Autodesk Inventor part; units mm, degrees
ref_plane "YZ Plane" through (0, 0, 0) normal (1, 0, 0) x (0, 1, 0)
ref_plane "XZ Plane" through (0, 0, 0) normal (0, 1, 0) x (-1, 0, 0)
ref_plane "XY Plane" through (0, 0, 0) normal (0, 0, 1) x (1, 0, 0)
sketch "Sketch1" plane through (0, 0, 0) normal (0, 0, 1) x (1, 0, 0)
  line L0 (0, 0) -> (97, 0)
  line L1 (97, 0) -> (97, 65)
  line L2 (97, 65) -> (0, 65)
  line L3 (0, 65) -> (0, 0)
  circle A0 centre (48.5, 32.5) radius 3
  line L4 (63.5, 47.5) -> (61.5, 47.5)
  line L5 (61.5, 47.5) -> (61.5, 17.5)
  line L6 (61.5, 17.5) -> (63.5, 17.5)
  line L7 (63.5, 17.5) -> (63.5, 47.5)
  line L8 (33.5, 47.5) -> (35.5, 47.5)
  line L9 (35.5, 47.5) -> (35.5, 17.5)
  line L10 (35.5, 17.5) -> (33.5, 17.5)
  line L11 (33.5, 17.5) -> (33.5, 47.5)
  line L12 (35.5, 49.5718) -> (61.5, 49.5718)
  line L13 (61.5, 49.5718) -> (61.5, 47.5718)
  line L14 (61.5, 47.5718) -> (35.5, 47.5718)
  line L15 (35.5, 47.5718) -> (35.5, 49.5718)
  line L16 (48.5, 32.5) -> (31.2053, 32.5)
  line L17 (31.2053, 32.5) -> (48.5, 32.5)
  line L18 (48.5, 32.5) -> (67.3058, 32.5)
  line L19 (35.5, 15.4282) -> (61.5, 15.4282)
  line L20 (61.5, 17.4282) -> (35.5, 17.4282)
  line L21 (61.5, 15.4282) -> (61.5, 17.4282)
  line L22 (35.5, 15.4282) -> (35.5, 17.4282)
  point P0 (0, 32.5)
  point P1 (62.5, 47.5)
  dimension "d2" = 97
  dimension "d3" = 65
  dimension "d4" = 6
  dimension "d6" = 32.5
  dimension "d7" = 48.5
  dimension "d8" = 2
  dimension "d9" = 30
  dimension "d12" = 15
  dimension "d13" = 2
  dimension "d14" = 30
  dimension "d15" = 15
  dimension "d16" = 2
  dimension "d20" = 26
  dimension "d21" = 0
extrude "Extrusion1" add sketch "Sketch1" along normal mid plane 1.8
Geometry check sheet. Reference: the model listing, model coordinates, mm. A direction names the side the tool comes from. Give positions to 0.01 mm unless a question says otherwise; leave off trailing zeros. Loops run counter-clockwise (first coordinate to the right, second up) from the corner with the lowest first, then second, coordinate; pieces in that order, holes last. Notation, with made-up numbers: M 55.25,-6 L 98.25,-6 A20 ccw 98.25,19 Z; hole C -19.75,54 d2. An arc over 180 degrees is marked long. Write item = value, one per line.
(1) Sectioned sample at A-A, the plane y = 28. Record the cut outline in (x, z).
Answer below:
outline = M 0,-0.9 L 33.5,-0.9 L 33.5,0.9 L 0,0.9 Z; M 35.5,-0.9 L 61.5,-0.9 L 61.5,0.9 L 35.5,0.9 Z; M 63.5,-0.9 L 97,-0.9 L 97,0.9 L 63.5,0.9 Z
(2) Release check for a two-part mould opening along X. For faces 1 (the face through (61.5, 49, 0)), 2 (the face through (0, 33, 0)), 3 (the face through (48, 0, 0)) record: released by +X, released by -X, zero draft, split by the parting line, or undercut.
Answer below:
face_1 = undercut
face_2 = released by -X
face_3 = zero draft
(3) Material ranges on line 1 (Y direction, x = 43, z = 0.6); line 2 (Y direction, x = 48.5, z = -0.1); line 3 (X direction, y = 46, z = -0.15), recorded low to high. Write a range as [from, to].
Answer below:
line_1 = [0, 15.43], [17.43, 47.57], [49.57, 65]
line_2 = [0, 15.43], [17.43, 29.5], [35.5, 47.57], [49.57, 65]
line_3 = [0, 33.5], [35.5, 61.5], [63.5, 97]
(4) Sectioned sample at B-B, the plane z = 0.4. Record the cut outline in (x, y), plus the area to 3 significant figures.
Answer below:
outline = M 0,0 L 97,0 L 97,65 L 0,65 Z; hole M 33.5,17.5 L 35.5,17.5 L 35.5,47.5 L 33.5,47.5 Z; hole M 35.5,15.43 L 61.5,15.43 L 61.5,17.43 L 35.5,17.43 Z; hole M 35.5,47.57 L 61.5,47.57 L 61.5,49.57 L 35.5,49.57 Z; hole C 48.5,32.5 d6; hole M 61.5,17.5 L 63.5,17.5 L 63.5,47.5 L 61.5,47.5 Z
area = 6,050 mm2
(5) Sectioned sample at C-C, the plane x = 48.5. Record the cut outline in (y, z).
Answer below:
outline = M 0,-0.9 L 15.43,-0.9 L 15.43,0.9 L 0,0.9 Z; M 17.43,-0.9 L 29.5,-0.9 L 29.5,0.9 L 17.43,0.9 Z; M 35.5,-0.9 L 47.57,-0.9 L 47.57,0.9 L 35.5,0.9 Z; M 49.57,-0.9 L 65,-0.9 L 65,0.9 L 49.57,0.9 Z
(6) Tool access check on faces 4 (the face through (49, 47.572, 0)), 5 (the face through (48, 40, -0.9)). Record the directions out of +Z, -Z, +X, -X, +Y, -Y that give a thin tool (end or side, any length) a straight path to the whole face; none if there is none.
Answer below:
face_4 = +Z, -Z
face_5 = -Z, +X, -X, +Y, -Y
